from build123d import *

# Parameters (mm, degrees)
SCHIZZO1_W                   = 9
SCHIZZO1_H                   = 9
ESTRUSIONE_ESTRUSIONE1_DEPTH = 5.2
SCHIZZO2_W                   = 1.17
SCHIZZO2_H                   = 3.52
TAGLIO_ESTRUSIONE1_DEPTH     = 10
RACCORDO1_R                  = 0.2


with BuildPart() as part:
    # Schizzo1 → Estrusione-Estrusione1 (new body)
    with BuildSketch(Plane(origin=(0, 0, 0), x_dir=(1, 0, 0), z_dir=(0, 1, 0))):
        Rectangle(SCHIZZO1_W, SCHIZZO1_H)
    extrude(amount=ESTRUSIONE_ESTRUSIONE1_DEPTH)

    # Schizzo2 → Taglio-Estrusione1 (cut, through all)
    with BuildSketch(Plane.XY.offset(4.5)):
        with Locations((-3.051, 3.44)):
            Rectangle(SCHIZZO2_W, SCHIZZO2_H)
        with Locations((1.017, 3.44)):
            Rectangle(SCHIZZO2_W, SCHIZZO2_H)
        with Locations((3.051, 3.44)):
            Rectangle(SCHIZZO2_W, SCHIZZO2_H)
        with Locations((-1.017, 3.44)):
            Rectangle(SCHIZZO2_W, SCHIZZO2_H)
    extrude(amount=-TAGLIO_ESTRUSIONE1_DEPTH, mode=Mode.SUBTRACT)

    # Raccordo1
    raccordo1_edges = [part.edges().sort_by_distance(p)[0] for p in [
        (-4.5, 5.2, 0),
        (-3.636, 5.2, 0),
        (-2.466, 5.2, 0),
        (0.432, 5.2, 0),
        (1.602, 5.2, 0),
        (4.5, 5.2, 0),
        (2.466, 5.2, 0),
        (3.636, 5.2, 0),
        (-4.5, 0, 0),
        (4.5, 0, 0),
        (-1.602, 5.2, 0),
        (-0.432, 5.2, 0),
    ]]
    fillet(raccordo1_edges, radius=RACCORDO1_R)


solid = part.part
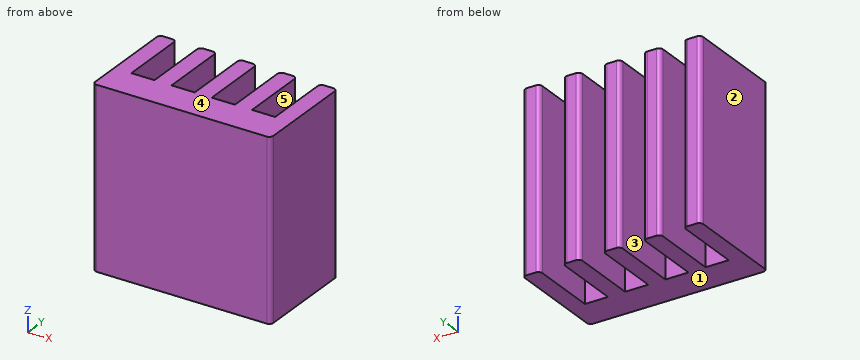
Part model, mm, in its own coordinate system. Face numbers are marked on the shaded views. A direction names the side the tool comes from. Round coordinates to 2 decimals unless told otherwise and drop trailing zeros. Loops run counter-clockwise (first coordinate to the right, second up) from the corner with the lowest first, then second, coordinate; pieces in that order, holes last. Notation, with made-up numbers: (55.5, -38) - (68.5, -38) arc R15 ccw to (68.5, -24) - close; hole circle Ø2 at (19, -22). An arc over 180 degrees is marked (long way). Answer as a JSON object with one key per item and string values.
Item 1: Tool access for the marked faces 4 and 5: list every direction of +Z, -Z, +X, -X, +Y, -Y with a clear straight run to the whole face (end or side of a thin tool).
Output:
{"face 4": "+Z, +X, -X, +Y, -Y", "face 5": "+Z, -Z, +Y"}
Item 2: Band-saw the part on C-C on x = -3. List the corners of the cut face in (y, z).
Output:
{"outline": "(0, -4.5) - (1.68, -4.5) - (1.68, 4.5) - (0, 4.5) - close"}
Item 3: Band-saw the part on B-B on y = 1.8. List the corners of the cut face in (x, z).
Output:
{"outline": "(-4.5, -4.5) - (-3.64, -4.5) - (-3.64, 4.5) - (-4.5, 4.5) - close; (-2.47, -4.5) - (-1.6, -4.5) - (-1.6, 4.5) - (-2.47, 4.5) - close; (-0.43, -4.5) - (0.43, -4.5) - (0.43, 4.5) - (-0.43, 4.5) - close; (1.6, -4.5) - (2.47, -4.5) - (2.47, 4.5) - (1.6, 4.5) - close; (3.64, -4.5) - (4.5, -4.5) - (4.5, 4.5) - (3.64, 4.5) - close"}
Item 4: Pin check, flat tips, straight feed: pin 1 (2 mm diameter, centred on x = 1.5, z = 2.5, fed in from +Y); pin 2 (0.6 mm diameter, centred on x = -1, z = -0.5, fed in from +Y). Stop position of each tip, or through.
Output:
{"pin 1": "y = 5.2", "pin 2": "y = 1.68"}
Item 5: Pull direction X, two halves, no side cores. Call the marked faces 1, 2 and 3: pulls with the +X half, pulls with the -X half, needs draft (parallel to the pull), parting line crosses it, or undercut.
Output:
{"face 1": "needs draft", "face 2": "pulls with the -X half", "face 3": "undercut"}
Item 6: Wall check: L1, parallel to X at y = 4.8, z = 2; L2, parallel to Y at x = -2.5, z = -1.75. Give the ranges that are in metal, low to high.
Output:
{"L1": "-4.5 to -3.64, -2.47 to -1.6, -0.43 to 0.43, 1.6 to 2.47, 3.64 to 4.5", "L2": "0 to 1.68"}
